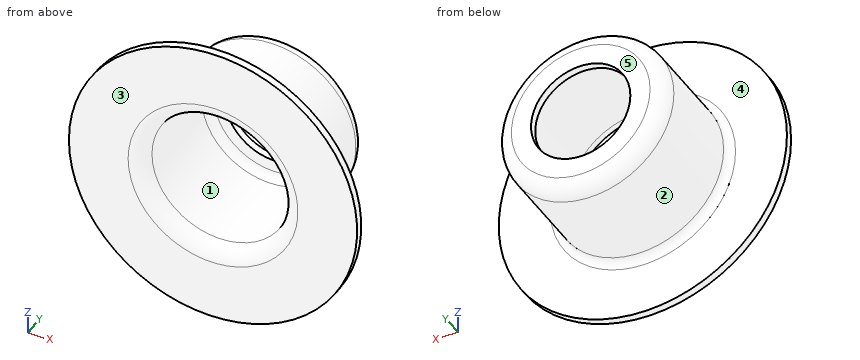
from build123d import *


with BuildPart() as part:
    # Sketch1 → Revolve1 (revolve)
    with BuildSketch(Plane.XY):
        with BuildLine():
            Line((-18.5, 0), (-10.9, 0))
            ThreePointArc((-10.9, 0), (-9.485786438, 0.585786438), (-8.9, 2))
            Line((-8.9, 2), (-8.9, 14))
            ThreePointArc((-8.9, 14), (-8.607106781, 14.707106781), (-7.9, 15))
            Line((-7.9, 15), (-6.375, 15))
            Line((-6.375, 15), (-6.375, 16))
            Line((-6.375, 16), (-8.9, 16))
            ThreePointArc((-8.9, 16), (-10.314213562, 15.414213562), (-10.9, 14))
            Line((-10.9, 14), (-10.9, 2))
            ThreePointArc((-10.9, 2), (-11.192893219, 1.292893219), (-11.9, 1))
            Line((-11.9, 1), (-18.5, 1))
            Line((-18.5, 1), (-18.5, 0))
        make_face()
    revolve(axis=Axis((0, 0, 0), (0, 1, 0)))


solid = part.part
The listing builds one solid part. Answer for the finished solid, in the listing's coordinates (mm). Face numbers are marked on the shaded views. A direction names the side the tool comes from. Round coordinates to 2 decimals unless told otherwise and drop trailing zeros. Order: outer loops, then holes, each group sorted by start corner. A loop starts at its lowest first (then second) coordinate and runs counter-clockwise, first axis right, second up. Notation, with made-up numbers: (73.25, 43.25) -> (132.25, 43.25) arc R18 ccw to (132.25, 64.25) -> close; hole circle Ø4 at (-38.5, 38.5). An arc over 180 degrees is marked (long way). Put each result on its own line as item: value.
Q1. Section A-A, the plane z = 0 is taken. Write down the section's boundary in (x, y) (3 decimals).
Results list:
outline: (-18.5, 0) -> (-10.9, 0) arc R2 ccw to (-8.9, 2) -> (-8.9, 14) arc R1 cw to (-7.9, 15) -> (-6.375, 15) -> (-6.375, 16) -> (-8.9, 16) arc R2 ccw to (-10.9, 14) -> (-10.9, 2) arc R1 cw to (-11.9, 1) -> (-18.5, 1) -> close; (6.375, 15) -> (7.9, 15) arc R1 cw to (8.9, 14) -> (8.9, 2) arc R2 ccw to (10.9, 0) -> (18.5, 0) -> (18.5, 1) -> (11.9, 1) arc R1 cw to (10.9, 2) -> (10.9, 14) arc R2 ccw to (8.9, 16) -> (6.375, 16) -> close
Q2. Consider line 1 along Z through (x, y) = (0, 6.75); line 2 along Z through (x, y) = (-2, 1.5); line 3 along X through (y, z) = (14.5, -2). Determine where each line is inside the solid, lowest interval first.
Results list:
line 1: -10.9 to -8.9, 8.9 to 10.9
line 2: -10.85 to -8.74, 8.74 to 10.85
line 3: -10.65 to -8.53, 8.53 to 10.65
Q3. Determine the mould class of the marked faces 1, 2 and 3 for opening direction Z: pulls with the +Z half, pulls with the -Z half, needs draft (parallel to the pull), parting line crosses it, or undercut.
Results list:
face 1: undercut
face 2: parting line crosses it
face 3: needs draft
Q4. Which of the six approach directions +Z, -Z, +X, -X, +Y, -Y give full straight-line access (tool end or side, diameter ignored) to the marked faces 4 and 5?
Results list:
face 4: +Y
face 5: +Z, -Z, +X, -X, +Y
Q5. Section B-B, the plane x = 0 is taken. Write down the section's boundary in (y, z) (3 decimals).
Results list:
outline: (0, -18.5) -> (1, -18.5) -> (1, -11.9) arc R1 cw to (2, -10.9) -> (14, -10.9) arc R2 ccw to (16, -8.9) -> (16, -6.375) -> (15, -6.375) -> (15, -7.9) arc R1 cw to (14, -8.9) -> (2, -8.9) arc R2 ccw to (0, -10.9) -> close; (0, 10.9) arc R2 ccw to (2, 8.9) -> (14, 8.9) arc R1 cw to (15, 7.9) -> (15, 6.375) -> (16, 6.375) -> (16, 8.9) arc R2 ccw to (14, 10.9) -> (2, 10.9) arc R1 cw to (1, 11.9) -> (1, 18.5) -> (0, 18.5) -> close
Q6. Section C-C, the plane y = 7.5 is taken. Write down the section's boundary in (x, z), and give its area (3 significant figures).
Results list:
outline: circle Ø21.8 at (0, 0); hole circle Ø17.8 at (0, 0)
area: 124 mm^2
Q7. Each of these flat-tipped pins is pushed along its axis until it touches: P1, Ø10, axis at x = 14, z = -9.5, coming from the +Y side; P2, Ø1.5, axis at x = -9, y = 8, coming from the -Z side; P3, Ø3, axis at y = 12, z = -11, coming from the -X side. Where does it stop, or does it pass through?
Results list:
P1: y = 1
P2: z = -7.12
P3: x = -5.34
